The listing builds one solid part. Answer for the finished solid, in the listing's coordinates (mm). A direction names the side the tool comes from. Give positions to 0.01 mm unless a question says otherwise; leave off trailing zeros. Order: outer loops, then holes, each group sorted by start corner. A loop starts at its lowest first (then second) coordinate and runs counter-clockwise, first axis right, second up. Notation, with made-up numbers: (52.25, 75.25) - (85.25, 75.25) arc R37 cw to (85.25, 113.25) - close; hole circle Ø5 at (44.5, 31.5). An arc over 180 degrees is marked (long way). Answer as a JSON object with one key per item and string values. Group by question number.
Q1. For faces 4 (the face through (-18.305, -6.342, -8.468)), 5 (the face through (-20.337, -3.226, -9.311)), 6 (the face through (0.2, -17.7, -9.9)), 7 (the face through (17.073, -5.523, -5.171)), 8 (the face through (-19, -1.5, -10)), determine the directions among +Z, -Z, +X, -X, +Y, -Y from which every point of the face is accessible in a straight line to the end or side of a thin tool.
Q2. A cutting plane is placed at B-B, the plane y = 0. Give the vertices of the cut face in (x, z), and give its area (3 significant figures).
Q3. A cutting plane is placed at A-A, the plane x = -22. Give the vertices of the cut face in (y, z).
Q4. Given pin 1 (6 mm diameter, centred on y = 0.5, z = -2.5, fed in from +X); pin 2 (4 mm diameter, centred on x = -21, z = -11, fed in from -Y); pin 3 (1.5 mm diameter, centred on y = -10, z = -13.5, fed in from +X); pin 4 (2 mm diameter, centred on x = 18, y = 0, fed in from -Z), each flat-ended and moving along its own axis, determine where each tip first touches the part or whether it passes through.
Q5. Consider line 1 (Y direction, x = 18, z = -18.65); line 2 (Z direction, x = -22, y = -3.7); line 3 (Z direction, x = -22, y = -5.75). Determine where each line is inside the solid, lowest interval first.
Q6. A cutting plane is placed at D-D, the plane y = 3.5. Give the vertices of the cut face in (x, z), and give its area (3 significant figures).
Q7. The mould has two halves that part along X. Classify faces 1 (the face through (-27, -6.5, -10)), 2 (the face through (14, 0, -18)), 3 (the face through (22.7, -4, -10)): released by +X, released by -X, zero draft, split by the parting line, or undercut.
Q8. A cutting plane is placed at C-C, the plane x = 18. Give the vertices of the cut face in (y, z), and give its area (3 significant figures).
from build123d import *

# Parameters (mm, degrees)
CYLINDER010_R     = 5.6
CYLINDER010_DEPTH = 10.2
CYLINDER007_R     = 4
CYLINDER007_DEPTH = 20
CYLINDER006_R     = 1.8
CYLINDER006_DEPTH = 20
CYLINDER001_R     = 4
CYLINDER001_DEPTH = 20
CYLINDER_R        = 1.8
CYLINDER_DEPTH    = 20
PAD_DEPTH         = 20
PAD001_DEPTH      = 5
CYLINDER009_R     = 5
CYLINDER009_DEPTH = 9.8


with BuildPart() as horizontal_body_space:
    # Cylinder010 → Cylinder010 (new body)
    with BuildSketch(Plane(origin=(18, 0, 9.8), x_dir=(1, 0, 0), z_dir=(0, 0, 1))):
        Circle(CYLINDER010_R)
    extrude(amount=CYLINDER010_DEPTH)


with BuildPart() as part_mirroring002:
    # Part__Mirroring002: instance of horizontal body space
    add(horizontal_body_space.part.mirror(Plane(origin=(0, 0, 10), x_dir=(0, 1, 0), z_dir=(0, 0, 1))))


with BuildPart() as horizontal_bolt_head_hole:
    # Cylinder007 → Cylinder007 (new body)
    with BuildSketch(Plane.XY.offset(17)):
        Circle(CYLINDER007_R)
    extrude(amount=CYLINDER007_DEPTH)


with BuildPart() as horizontal_bolt_hole_fusion:
    # Cylinder006 → Cylinder006 (new body)
    with BuildSketch(Plane.XY):
        Circle(CYLINDER006_R)
    extrude(amount=CYLINDER006_DEPTH)

    # Fusion003: union horizontal bolt head hole
    add(horizontal_bolt_head_hole.part)


with BuildPart() as horizontal_bolt_hole_fusion_1:
    # Fusion003 placement: moved
    add(horizontal_bolt_hole_fusion.part.moved(Location((18, 0, 0))))


with BuildPart() as bolt_head_hole:
    # Cylinder001 → Cylinder001 (new body)
    with BuildSketch(Plane.XZ):
        Circle(CYLINDER001_R)
    extrude(amount=CYLINDER001_DEPTH)


with BuildPart() as fusion005:
    # Cylinder → Cylinder (new body)
    with BuildSketch(Plane.XZ.offset(-10)):
        Circle(CYLINDER_R)
    extrude(amount=CYLINDER_DEPTH)

    # Fusion: union bolt head hole
    add(bolt_head_hole.part)


with BuildPart() as fusion005_1:
    # Fusion placement: moved
    add(fusion005.part.moved(Location((-22, -5, 10))))

    # Fusion005: union Part__Mirroring002, horizontal bolt hole fusion
    add(part_mirroring002.part)
    add(horizontal_bolt_hole_fusion_1.part)


with BuildPart() as f_25_mm_attachment_body:
    # Sketch → Pad (new body)
    with BuildSketch(Plane.XY):
        with BuildLine():
            ThreePointArc((12.611106, 1.5), (0, 12.7), (-12.611106, 1.5))
            Line((-22.7, 1.5), (-12.611106, 1.5))
            Line((-22.7, 1.5), (-22.7, 6.5))
            Line((-22.7, 6.5), (-21.463293, 6.5))
            Line((-21.463293, 6.5), (-13.988671, 10.84468))
            ThreePointArc((13.988671, 10.84468), (0, 17.7), (-13.988671, 10.84468))
            Line((13.988671, 10.84468), (21.463293, 6.5))
            Line((21.463293, 6.5), (22.7, 6.5))
            Line((22.7, 6.5), (22.7, 1.5))
            Line((12.611106, 1.5), (22.7, 1.5))
        make_face()
    extrude(amount=PAD_DEPTH)

    # Sketch001 → Pad001 (join)
    with BuildSketch(Plane.XZ.offset(-1.5)):
        with BuildLine():
            Line((-12.611106, 20), (-22.7, 20))
            ThreePointArc((-22.7, 20), (-27.649747, 17.949747), (-29.7, 13))
            Line((-29.7, 13), (-29.7, 7))
            ThreePointArc((-29.7, 7), (-27.649747, 2.050253), (-22.7, 0))
            Line((-12.611106, 0), (-22.7, 0))
            Line((-12.611106, 20), (-12.611106, 0))
        make_face()
    extrude(amount=-PAD001_DEPTH)


with BuildPart() as part_mirroring:
    # Part__Mirroring: instance of 25 mm attachment body
    add(f_25_mm_attachment_body.part.mirror(Plane(origin=(0, 0, 0), x_dir=(1, 0, 0), z_dir=(0, 1, 0))))


with BuildPart() as horizontal_body:
    # Cylinder009 → Cylinder009 (new body)
    with BuildSketch(Plane(origin=(18, 0, 0), x_dir=(1, 0, 0), z_dir=(0, 0, 1))):
        Circle(CYLINDER009_R)
    extrude(amount=CYLINDER009_DEPTH)


with BuildPart() as f_25_mm_attachment_holed_clone:
    # Part__Mirroring001: instance of horizontal body
    add(horizontal_body.part.mirror(Plane(origin=(0, 0, 10), x_dir=(0, 1, 0), z_dir=(0, 0, 1))))

    # Fusion004: union Part__Mirroring
    add(part_mirroring.part)

    # Cut: cut Fusion005
    add(fusion005_1.part, mode=Mode.SUBTRACT)


with BuildPart() as part_mirroring004:
    # Part__Mirroring004: instance of 25 mm attachment holed clone
    add(f_25_mm_attachment_holed_clone.part.mirror(Plane(origin=(0, 0, 0), x_dir=(0, 1, 0), z_dir=(0, 0, 1))))


solid = part_mirroring004.part
Reply:
{
 "1": {"face 4": "-Y", "face 5": "+Y, -Y", "face 6": "+Z, -Z, -Y", "face 7": "+Z, +Y", "face 8": "+Z, -Z, -X, +Y"},
 "2": {"outline": "(13, -20) - (14, -20) - (14, -17) - (16.2, -17) - (16.2, -10.2) - (13, -10.2) - close; (19.8, -17) - (22, -17) - (22, -20) - (23, -20) - (23, -10.2) - (19.8, -10.2) - close", "area": "49.5 mm^2"},
 "3": {"outline": "(-6.5, -20) - (-1.5, -20) - (-1.5, -11.8) - (-5, -11.8) - (-5, -14) - (-6.5, -14) - close; (-6.5, -6) - (-5, -6) - (-5, -8.2) - (-1.5, -8.2) - (-1.5, 0) - (-6.5, 0) - close"},
 "4": {"pin 1": "stops at x = 12.99", "pin 2": "stops at y = -5", "pin 3": "stops at x = 16.73", "pin 4": "passes through"},
 "5": {"line 1": "y = -8.51 to -4, 4 to 5", "line 2": "z = -20 to -11.8, -8.2 to 0", "line 3": "z = -20 to -14, -6 to 0"},
 "6": {"outline": "(14.43, -20) - (16.06, -20) - (16.06, -17) - (19.94, -17) - (19.94, -20) - (21.57, -20) - (21.57, -10.2) - (14.43, -10.2) - close", "area": "58.4 mm^2"},
 "7": {"face 1": "zero draft", "face 2": "undercut", "face 3": "released by +X"},
 "8": {"outline": "(-8.51, -20) - (-4, -20) - (-4, -17) - (-1.8, -17) - (-1.8, -10.2) - (-5.6, -10.2) - (-5.6, 0) - (-8.51, 0) - close; (1.8, -17) - (4, -17) - (4, -20) - (5, -20) - (5, -10.2) - (1.8, -10.2) - close", "area": "114 mm^2"}
}
